Here's how the part is built. I have some questions about the finished solid (model axes, mm). Face numbers are marked on the shaded views. A direction names the side the tool comes from. Round coordinates to 2 decimals unless told otherwise and drop trailing zeros. Loops run counter-clockwise (first coordinate to the right, second up) from the corner with the lowest first, then second, coordinate; pieces in that order, holes last. Notation, with made-up numbers: M 44.25,65 L 90.25,65 A19 ccw 90.25,93 Z; hole C -4.75,35 d8. An arc over 180 degrees is marked long. Answer as CSV lines item,"result".
```python
from build123d import *

# Parameters (mm, degrees)
PAD004_DEPTH = 23.5
PAD003_DEPTH = 23.5
SKETCH004_R  = 1.7
PAD002_DEPTH = 32.5
SKETCH003_R  = 1.7
PAD001_DEPTH = 32.5
SKETCH_R     = 30
SKETCH_R_2   = 20
PAD_DEPTH    = 7.5
SKETCH001_R  = 2.2
POCKET_DEPTH = 15.001
FILLET_R     = 1


with BuildPart() as pad_m3nut1:
    # Sketch006 → Pad004 (new body, symmetric)
    with BuildSketch(Plane.XZ):
        Polygon((1.587713, -2.75), (3.175426, 0), (1.587713, 2.75), (-1.587713, 2.75), (-3.175426, 0), (-1.587713, -2.75), align=None)
    extrude(amount=PAD004_DEPTH, both=True)


with BuildPart() as pad_m3nut:
    # Sketch005 → Pad003 (new body, symmetric)
    with BuildSketch(Plane.YZ):
        Polygon((3.175426, 0), (1.587713, 2.75), (-1.587713, 2.75), (-3.175426, 0), (-1.587713, -2.75), (1.587713, -2.75), align=None)
    extrude(amount=PAD003_DEPTH, both=True)


with BuildPart() as pad_m3_pocket1:
    # Sketch004 → Pad002 (new body, symmetric)
    with BuildSketch(Plane.YZ):
        Circle(SKETCH004_R)
    extrude(amount=PAD002_DEPTH, both=True)


with BuildPart() as pad_m3_pocket2:
    # Sketch003 → Pad001 (new body, symmetric)
    with BuildSketch(Plane.XZ):
        Circle(SKETCH003_R)
    extrude(amount=PAD001_DEPTH, both=True)


with BuildPart() as fillet_body:
    # Sketch → Pad (new body, symmetric)
    with BuildSketch(Plane.XY):
        Circle(SKETCH_R)
        Circle(SKETCH_R_2, mode=Mode.SUBTRACT)
    extrude(amount=PAD_DEPTH, both=True)

    # Sketch001 (on Face4 of Pad) → Pocket (cut, through all)
    with BuildSketch(Plane.XY.offset(7.5)):
        with Locations((-17.67767, 17.67767)):
            Circle(SKETCH001_R)
        with Locations((17.67767, 17.67767)):
            Circle(SKETCH001_R)
        with Locations((-17.67767, -17.67767)):
            Circle(SKETCH001_R)
        with Locations((17.67767, -17.67767)):
            Circle(SKETCH001_R)
    extrude(amount=-POCKET_DEPTH, mode=Mode.SUBTRACT)

    # Cut: cut Pad-M3-pocket2
    add(pad_m3_pocket2.part, mode=Mode.SUBTRACT)

    # Cut001: cut Pad-M3-pocket1
    add(pad_m3_pocket1.part, mode=Mode.SUBTRACT)

    # Cut002: cut Pad-M3Nut
    add(pad_m3nut.part, mode=Mode.SUBTRACT)

    # Cut003: cut Pad-M3Nut1
    add(pad_m3nut1.part, mode=Mode.SUBTRACT)

    # Fillet
    fillet_edges = [fillet_body.edges().sort_by_distance(p)[0] for p in [
        (-30, 0, 7.5),
        (-30, 0, -7.5),
        (-20, 0, 7.5),
        (-20, 0, -7.5),
    ]]
    fillet(fillet_edges, radius=FILLET_R)


solid = fillet_body.part
```
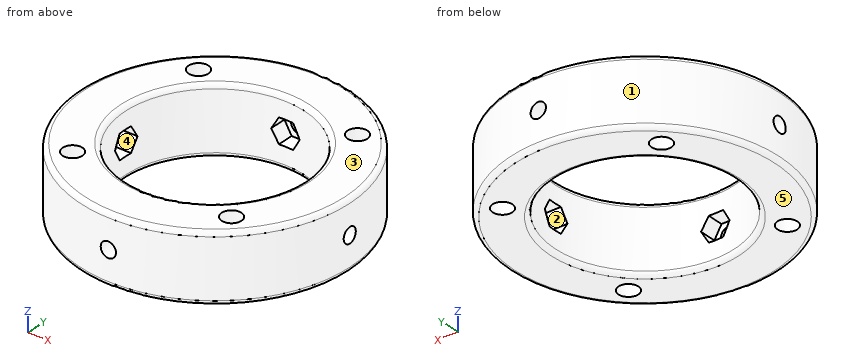
1. Which directions (+Z, -Z, +X, -X, +Y, -Y) give clear straight access to the entire face, cutting with the end or side of a thin tool? Please do the marked faces 1 and 2.
Evaluation:
face 1,"+Z, -Z"
face 2,"none"
2. I want a section at C-C, the plane z = 4. Please give me the cut outline in (x, y), and give its area (3 significant figures).
Evaluation:
outline,"C 0,0 d60; hole C 0,0 d40; hole C -17.68,-17.68 d4.4; hole C -17.68,17.68 d4.4; hole C 17.68,-17.68 d4.4; hole C 17.68,17.68 d4.4"
area,"1,510 mm²"
3. If I drill on line 1 (Y direction, x = -1, z = -2.5); line 2 (X direction, y = -17.5, z = 3.5); line 3 (Y direction, x = -16.5, z = -2.5), over which ranges is the centre line in solid material (lowest first)? Write a range as [from, to].
Evaluation:
line 1,"y = [-29.98, -23.5], [23.5, 29.98]"
line 2,"x = [-24.37, -19.87], [-15.48, -9.68], [9.68, 15.48], [19.87, 24.37]"
line 3,"y = [-25.05, -19.54], [-15.82, -11.3], [11.3, 15.82], [19.54, 25.05]"
4. For P1, Ø8, axis at y = 4.5, z = -2.5, coming from the -X side; P2, Ø4, axis at x = -10, z = 1, coming from the -Y side; P3, Ø4, axis at x = 10.5, z = 1, coming from the +Y side; P4, Ø4, axis at x = -17.68, y = -17.68, coming from the +Z side, each with a flat end and sliding along its axis, tell me the tip position at first contact or that it passes through.
Evaluation:
P1,"stops at x = -30"
P2,"stops at y = -28.91"
P3,"stops at y = 28.77"
P4,"passes through"
5. I want a section at A-A, the plane y = 0. Count the separate pieces of the cut face and the enclosed holes in it, and give its area (3 significant figures).
Evaluation:
separate pieces,"4"
enclosed holes,"0"
area,"216 mm²"
6. We'd pull the mould along Z, two halves only. Please class the marked faces 3, 4 and 5: pulls with the +Z half, pulls with the -Z half, needs draft (parallel to the pull), parting line crosses it, or undercut.
Evaluation:
face 3,"pulls with the +Z half"
face 4,"undercut"
face 5,"pulls with the -Z half"
